Answer from the drawing. Dimensions are ordinates in mm from the lowest x, y and z of the part. A direction names the side the tool comes from. Give positions to 0.01 mm unless a question says otherwise; leave off trailing zeros. Order: outer loops, then holes, each group sorted by start corner. A loop starts at its lowest first (then second) coordinate and runs counter-clockwise, first axis right, second up.
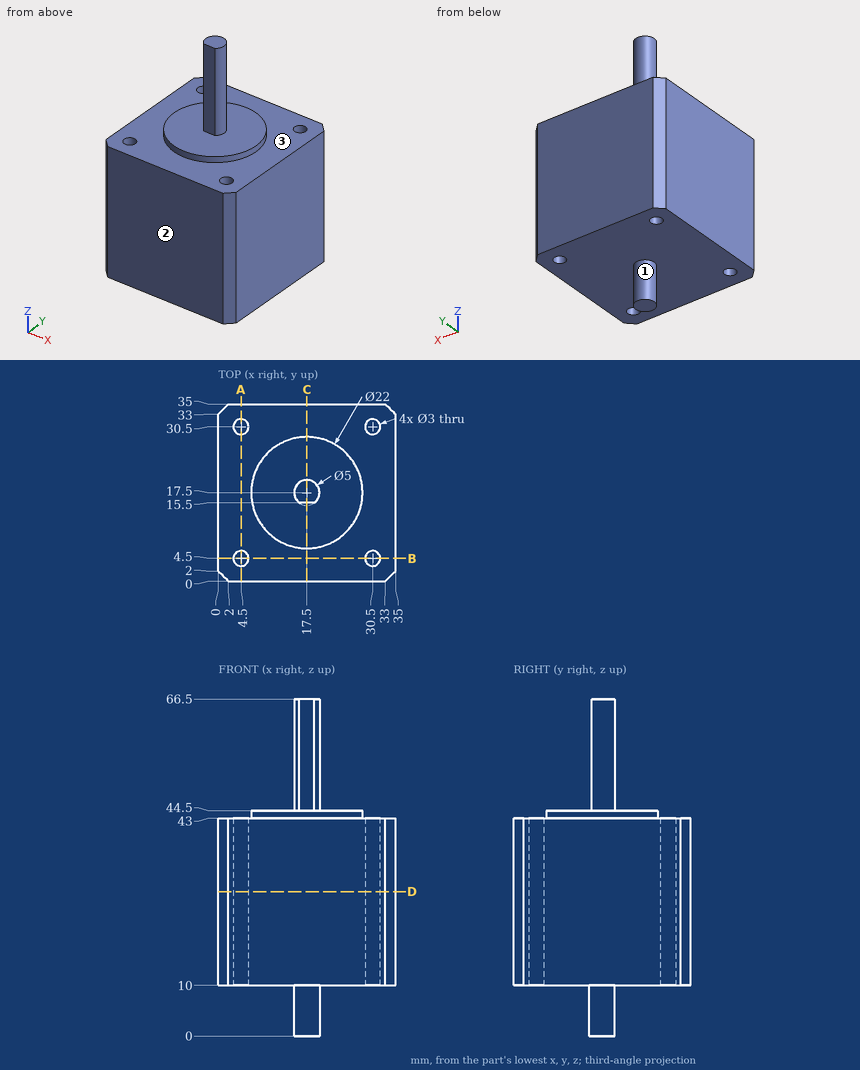
1. The part is cut by section C-C (x = 17.5). Write down the section's boundary in (y, z).
Findings below:
outline: (0, 10) - (15, 10) - (15, 0) - (20, 0) - (20, 10) - (35, 10) - (35, 43) - (28.5, 43) - (28.5, 44.5) - (20, 44.5) - (20, 66.5) - (15.5, 66.5) - (15.5, 44.5) - (6.5, 44.5) - (6.5, 43) - (0, 43) - close
2. Given P1, Ø1, axis at x = 18.5, z = 52.5, coming from the +Y side; P2, Ø6, axis at y = 11, z = 15, coming from the -X side; P3, Ø5, axis at x = 30.5, y = 4.5, coming from the +Z side; P4, Ø2.5, axis at x = 17, z = 55, coming from the -Y side, each flat-ended and moving along its own axis, determine where each tip first touches the part or whether it passes through.
Findings below:
P1: stops at y = 19.95
P2: stops at x = 0
P3: stops at z = 43
P4: stops at y = 15.5
3. Straight lines are drawn through the part: probe 1 along Y at (x, z) = (4.5, 26); probe 2 along Z at (x, y) = (9, 22.5); probe 3 along Z at (x, y) = (2, 2). For each, find the intervals that lie inside material, in ascending order.
Findings below:
probe 1: y = 0 to 3, 6 to 29, 32 to 35
probe 2: z = 10 to 44.5
probe 3: z = 10 to 43
4. The part is cut by section D-D (z = 28.5). Write down the section's boundary in (x, y), then the cut area to 3 significant figures.
Findings below:
outline: (0, 2) - (2, 0) - (33, 0) - (35, 2) - (35, 33) - (33, 35) - (2, 35) - (0, 33) - close; hole circle Ø3 at (4.5, 4.5); hole circle Ø3 at (4.5, 30.5); hole circle Ø3 at (30.5, 4.5); hole circle Ø3 at (30.5, 30.5)
area: 1,190 mm2
5. Which of the six approach directions +Z, -Z, +X, -X, +Y, -Y give full straight-line access (tool end or side, diameter ignored) to the marked faces 1, 2 and 3?
Findings below:
face 1: -Z
face 2: +Z, -Z, +X, -X, -Y
face 3: +Z
6. The part is cut by section A-A (x = 4.5). Write down the section's boundary in (y, z), then the cut area to 3 significant figures.
Findings below:
outline: (0, 10) - (3, 10) - (3, 43) - (0, 43) - close; (6, 10) - (29, 10) - (29, 43) - (6, 43) - close; (32, 10) - (35, 10) - (35, 43) - (32, 43) - close
area: 957 mm2
